Autodesk Inventor part; units mm, degrees
ref_plane "YZ Plane" through (0, 0, 0) normal (1, 0, 0) x (0, 1, 0)
ref_plane "XZ Plane" through (0, 0, 0) normal (0, 1, 0) x (-1, 0, 0)
ref_plane "XY Plane" through (0, 0, 0) normal (0, 0, 1) x (1, 0, 0)
sketch "Sketch1" plane through (0, 0, 0) normal (0, 1, 0) x (-1, 0, 0)
  line L0 (50, 75) -> (-50, 75)
  line L1 (-50, 75) -> (-50, -75)
  line L2 (-50, -75) -> (50, -75)
  line L3 (50, -75) -> (50, 75)
  line L4 (50, 75) -> (-50, -75) construction
  line L5 (-50, 75) -> (50, -75) construction
  circle A0 centre (0, 59.5) radius 2
  line L6 (0, 0) -> (50, 0) construction
  circle A1 centre (0, -59.5) radius 2
  dimension "d0" = 150
  dimension "d1" = 100
  dimension "d2" = 59.5
  dimension "d3" = 4
extrude "Extrusion1" add sketch "Sketch1" along normal blind 10
fillet "Fillet1" radius 5 4 edges at (50, 5, 75) (50, 5, -75) (-50, 5, 75) (-50, 5, -75)
sketch "Sketch2" plane through (0, 10, 0) normal (0, 1, 0) x (1, 0, 0)
  line L0 (-40, -47.5) -> (40, -47.5)
  line L1 (40, -47.5) -> (40, 47.5)
  line L2 (40, 47.5) -> (-40, 47.5)
  line L3 (-40, 47.5) -> (-40, -47.5)
  line L4 (-40, -47.5) -> (40, 47.5) construction
  line L5 (40, -47.5) -> (-40, 47.5) construction
  point P0 (0, 0)
  dimension "d7" = 95
  dimension "d8" = 80
extrude "Extrusion2" cut sketch "Sketch2" against normal blind 10
fillet "Fillet2" radius 5 4 edges at (-40, 5, -47.5) (40, 5, -47.5) (40, 5, 47.5) (-40, 5, 47.5)
properties part number "Base(4mm holes)"
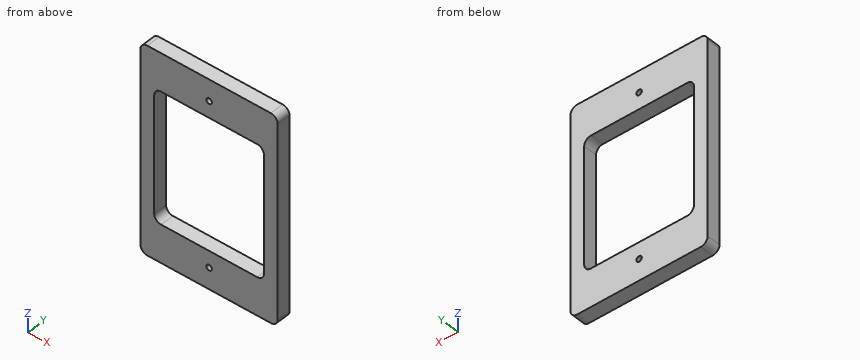
CAD build for the part. Positions are in the model's coordinates, mm. Give positions to 0.01 mm unless a question says otherwise; leave off trailing zeros. Write each loop counter-clockwise with the first axis right and the second up, starting at its lowest first coordinate (ties: lowest second). Pieces come first, ordered by that corner, then holes. Notation, with made-up numbers: M 56,-26.5 L 114,-26.5 A13 ccw 114,-21.5 Z; hole C 88,50 d8. An arc over 180 degrees is marked long. Put each result on its own line as item: value. Start each with the question number.
(1) Probe L1, parallel to Z at x = 0, y = 4.5; L2, parallel to X at y = 5.25, z = -2; L3, parallel to Z at x = 20.5, y = 2.25. List the from-to ranges inside material, lowest first.
(2) Band-saw the part on C-C, the plane y = 3. Write the cut outline in (x, z), and give its area (3 significant figures).
(3) Band-saw the part on A-A, the plane x = 0. Write the cut outline in (y, z).
(4) Band-saw the part on B-B, the plane z = 59.5. Write the cut outline in (x, y).
(5) Band-saw the part on D-D, the plane x = 28. Write the cut outline in (y, z).
Response values:
1. L1: z = -75 to -61.5, -57.5 to -47.5, 47.5 to 57.5, 61.5 to 75
1. L2: x = -50 to -40, 40 to 50
1. L3: z = -75 to -47.5, 47.5 to 75
2. outline: M -50,-70 A5 ccw -45,-75 L 45,-75 A5 ccw 50,-70 L 50,70 A5 ccw 45,75 L -45,75 A5 ccw -50,70 Z; hole M -40,-42.5 A5 ccw -35,-47.5 L 35,-47.5 A5 ccw 40,-42.5 L 40,42.5 A5 ccw 35,47.5 L -35,47.5 A5 ccw -40,42.5 Z; hole C 0,-59.5 d4; hole C 0,59.5 d4
2. area: 7,370 mm2
3. outline: M 0,-75 L 10,-75 L 10,-61.5 L 0,-61.5 Z; M 0,-57.5 L 10,-57.5 L 10,-47.5 L 0,-47.5 Z; M 0,47.5 L 10,47.5 L 10,57.5 L 0,57.5 Z; M 0,61.5 L 10,61.5 L 10,75 L 0,75 Z
4. outline: M -50,0 L -2,0 L -2,10 L -50,10 Z; M 2,0 L 50,0 L 50,10 L 2,10 Z
5. outline: M 0,-75 L 10,-75 L 10,-47.5 L 0,-47.5 Z; M 0,47.5 L 10,47.5 L 10,75 L 0,75 Z
